Autodesk Inventor part; units mm, degrees
ref_plane "YZ Plane" through (0, 0, 0) normal (1, 0, 0) x (0, 1, 0)
ref_plane "XZ Plane" through (0, 0, 0) normal (0, 1, 0) x (-1, 0, 0)
ref_plane "XY Plane" through (0, 0, 0) normal (0, 0, 1) x (1, 0, 0)
sketch "Sketch1" plane through (0, 0, 0) normal (0, 1, 0) x (-1, 0, 0)
  arc A0 (2.8605, 1.9692) -> (1.9692, 2.8605) centre (2.4696, 2.4696) ccw
  line L0 (1.3405, 2.2319) -> (1.9692, 2.8605)
  arc A1 (1.3405, 2.2319) -> (-1.3405, 2.2319) centre (0, 0) ccw
  line L1 (-1.9692, 2.8605) -> (-1.3405, 2.2319)
  arc A2 (-1.9692, 2.8605) -> (-2.8605, 1.9692) centre (-2.4696, 2.4696) ccw
  line L2 (-2.2319, 1.3405) -> (-2.8605, 1.9692)
  arc A3 (-2.2319, 1.3405) -> (-2.2319, -1.3405) centre (0, 0) ccw
  line L3 (-2.8605, -1.9692) -> (-2.2319, -1.3405)
  arc A4 (-2.8605, -1.9692) -> (-1.9692, -2.8605) centre (-2.4696, -2.4696) ccw
  line L4 (-1.3405, -2.2319) -> (-1.9692, -2.8605)
  arc A5 (-1.3405, -2.2319) -> (1.3405, -2.2319) centre (0, 0) ccw
  line L5 (1.9692, -2.8605) -> (1.3405, -2.2319)
  arc A6 (1.9692, -2.8605) -> (2.8605, -1.9692) centre (2.4696, -2.4696) ccw
  line L6 (2.2319, -1.3405) -> (2.8605, -1.9692)
  arc A7 (2.2319, -1.3405) -> (2.2319, 1.3405) centre (0, 0) ccw
  line L7 (2.8605, 1.9692) -> (2.2319, 1.3405)
  arc A8 (-4.5172, 1.6401) -> (-5.4471, 3.8852) centre (-7.6922, 1.6401) ccw
  line L8 (-8.7558, 7.1939) -> (-5.4471, 3.8852)
  arc A9 (-8.7558, 7.1939) -> (-10.4905, 6.4753) centre (-9.4743, 6.4753) ccw
  line L9 (-10.4905, -6.4748) -> (-10.4905, 6.4753)
  arc A10 (-10.4905, -6.4748) -> (-8.7558, -7.1933) centre (-9.4743, -6.4748) ccw
  line L10 (-5.4471, -3.8846) -> (-8.7558, -7.1933)
  arc A11 (-5.4471, -3.8846) -> (-4.5172, -1.6396) centre (-7.6922, -1.6396) ccw
  line L11 (-4.5172, 1.6401) -> (-4.5172, -1.6396)
  arc A12 (1.6396, 4.5172) -> (3.8846, 5.4471) centre (1.6396, 7.6922) ccw
  line L12 (3.8846, 5.4471) -> (7.1933, 8.7558)
  arc A13 (7.1933, 8.7558) -> (6.4748, 10.4905) centre (6.4748, 9.4743) ccw
  line L13 (6.4748, 10.4905) -> (4.356, 10.4905)
  arc A14 (4.356, 12.7003) -> (4.356, 10.4905) centre (4.356, 11.5954) ccw
  line L14 (4.356, 12.7003) -> (10.5919, 12.7003)
  arc A15 (12.7001, 10.5921) -> (10.5919, 12.7003) centre (10.5919, 10.5921) ccw
  line L15 (12.7001, 10.5921) -> (12.7001, 4.3562)
  arc A16 (10.4903, 4.3562) -> (12.7001, 4.3562) centre (11.5952, 4.3562) ccw
  line L16 (10.4903, 4.3562) -> (10.4903, 6.475)
  arc A17 (10.4903, 6.475) -> (8.7555, 7.1936) centre (9.4741, 6.475) ccw
  line L17 (8.7555, 7.1936) -> (5.4468, 3.8849)
  arc A18 (5.4468, 3.8849) -> (4.5169, 1.6399) centre (7.6919, 1.6399) ccw
  line L18 (4.5169, 1.6399) -> (4.5169, -1.6396)
  arc A19 (4.5169, -1.6396) -> (5.4468, -3.8846) centre (7.6919, -1.6396) ccw
  line L19 (5.4468, -3.8846) -> (8.7555, -7.1933)
  arc A20 (8.7555, -7.1933) -> (10.4903, -6.4748) centre (9.4741, -6.4748) ccw
  line L20 (10.4903, -6.4748) -> (10.4903, -4.356)
  arc A21 (12.7001, -4.356) -> (10.4903, -4.356) centre (11.5952, -4.356) ccw
  line L21 (12.7001, -4.356) -> (12.7001, -10.5919)
  arc A22 (10.5919, -12.7001) -> (12.7001, -10.5919) centre (10.5919, -10.5919) ccw
  line L22 (10.5919, -12.7001) -> (4.356, -12.7001)
  arc A23 (4.356, -10.4903) -> (4.356, -12.7001) centre (4.356, -11.5952) ccw
  line L23 (4.356, -10.4903) -> (6.475, -10.4903)
  arc A24 (6.475, -10.4903) -> (7.1936, -8.7555) centre (6.475, -9.4741) ccw
  line L24 (7.1936, -8.7555) -> (3.8846, -5.4465)
  arc A25 (3.8846, -5.4465) -> (1.6396, -4.5166) centre (1.6396, -7.6916) ccw
  line L25 (1.6396, -4.5166) -> (-1.6396, -4.5166)
  arc A26 (-1.6396, -4.5166) -> (-3.8846, -5.4465) centre (-1.6396, -7.6916) ccw
  line L26 (-3.8846, -5.4465) -> (-7.1936, -8.7555)
  arc A27 (-7.1936, -8.7555) -> (-6.475, -10.4903) centre (-6.475, -9.4741) ccw
  line L27 (-6.475, -10.4903) -> (-4.3562, -10.4903)
  arc A28 (-4.3562, -12.7001) -> (-4.3562, -10.4903) centre (-4.3562, -11.5952) ccw
  line L28 (-4.3562, -12.7001) -> (-10.5919, -12.7001)
  arc A29 (-12.7001, -10.5919) -> (-10.5919, -12.7001) centre (-10.5919, -10.5919) ccw
  line L29 (-12.7001, -10.5919) -> (-12.7001, 10.5921)
  arc A30 (-10.5919, 12.7003) -> (-12.7001, 10.5921) centre (-10.5919, 10.5921) ccw
  line L30 (-10.5919, 12.7003) -> (-4.3562, 12.7003)
  arc A31 (-4.3562, 10.4905) -> (-4.3562, 12.7003) centre (-4.3562, 11.5954) ccw
  line L31 (-4.3562, 10.4905) -> (-6.475, 10.4905)
  arc A32 (-6.475, 10.4905) -> (-7.1936, 8.7558) centre (-6.475, 9.4743) ccw
  line L32 (-7.1936, 8.7558) -> (-3.8849, 5.4471)
  arc A33 (-3.8849, 5.4471) -> (-1.6399, 4.5172) centre (-1.6399, 7.6922) ccw
  line L33 (-1.6399, 4.5172) -> (1.6396, 4.5172)
  point P0 (0, 0)
  dimension "d36" = 8.1835
  dimension "d81" = 1.0162
  dimension "d82" = 3.175
  dimension "d95" = 8.1832
  dimension "d96" = 17.2172
  dimension "d97" = 23.1906
  dimension "d98" = 25.4002
  dimension "d100" = 8.1832
  dimension "d101" = 2.2092
  dimension "d104" = 2.2091
  dimension "d131" = 1.1049
  dimension "d132" = 2.1082
  dimension "d133" = 0.635
  dimension "d134" = 2.6035
  dimension "d135" = 2.6035
  dimension "d136" = 2.6035
  dimension "d137" = 2.6035
  dimension "d138" = 45
  dimension "d139" = 45
  dimension "d140" = 45
  dimension "d141" = 45
  dimension "d142" = 45
  dimension "d143" = 25.4004
  dimension "d144" = 0.4742
  dimension "d145" = 1.7347
  dimension "d146" = 0.4744
  dimension "d147" = 1.7349
  dimension "d148" = 12.7001
  dimension "d149" = 12.7003
  dimension "d150" = 1.1046
  dimension "d151" = 1.1048
  dimension "d152" = 0.6303
  dimension "d153" = 0.6303
  dimension "d154" = 0.6303
  dimension "d155" = 0.6303
  dimension "d156" = 8.3441
  dimension "d157" = 17.0563
  dimension "d158" = 8.3441
  dimension "d159" = 8.3441
  dimension "d160" = 9.8396
  dimension "d161" = 9.8396
  dimension "d162" = 10.2305
  dimension "d163" = 10.2305
  dimension "d164" = 10.4682
  dimension "d165" = 10.4682
  dimension "d166" = 14.6692
  dimension "d167" = 14.6692
  dimension "d168" = 15.1696
  dimension "d169" = 15.1696
  dimension "d170" = 17.0563
  dimension "d171" = 17.0563
extrude "Extrusion1" add sketch "Sketch1" along normal mid plane 25.4
properties part number "1003-S-BLACK-FB" material "6105-T5"
The listing builds one solid part. Answer for the finished solid, in the listing's coordinates (mm). A direction names the side the tool comes from. Coordinates: 2 decimals unless noted, no trailing zeros. Write each loop counter-clockwise with the first axis right and the second up, starting at its lowest first coordinate (ties: lowest second). Pieces come first, ordered by that corner, then holes.
Q1. Section D-D, the plane y = 10.25 is taken. Give the number of separate pieces and of enclosed holes in the cut face, then the cut area to 3 significant figures.
Returned:
separate pieces: 1
enclosed holes: 2
area: 295 mm2
Q2. Given P1, Ø1, axis at x = 0, y = 2.5, coming from the +Z side; P2, Ø1, axis at x = -2.47, z = -2.47, coming from the -Y side; P3, Ø1.6, axis at y = 2.5, z = 0, coming from the -X side; P4, Ø1.6, axis at x = 0, y = -5, coming from the -Z side, each flat-ended and moving along its own axis, determine where each tip first touches the part or whether it passes through.
Returned:
P1: stops at z = 4.52
P2: passes through
P3: stops at x = -4.52
P4: stops at z = -4.52
Q3. Section C-C, the plane x = -5 is taken. Write down the section's boundary in (y, z), then the cut area to 3 significant figures.
Returned:
outline: (-12.7, -12.7) - (12.7, -12.7) - (12.7, -10.49) - (-12.7, -10.49) - close; (-12.7, -6.56) - (12.7, -6.56) - (12.7, -3.32) - (-12.7, -3.32) - close; (-12.7, 3.32) - (12.7, 3.32) - (12.7, 6.56) - (-12.7, 6.56) - close; (-12.7, 10.49) - (12.7, 10.49) - (12.7, 12.7) - (-12.7, 12.7) - close
area: 277 mm2
Q4. The mould has two halves that part along Z. Classify faces 3 (the cylindrical face through (2.871, -0.178, -4.765)), 4 (the flat face through (-8, 0, -12.7)), 5 (the cylindrical face through (-4.752, -0.178, 2.839)), 6 (the flat face through (-7, 0, 12.7)): released by +Z, released by -Z, zero draft, split by the parting line, or undercut.
Returned:
face 3: undercut
face 4: released by -Z
face 5: undercut
face 6: released by +Z
Q5. Section B-B, the plane z = 11 is taken. Write down the section's boundary in (x, y), then the cut area to 3 significant figures.
Returned:
outline: (-12.66, -12.7) - (-3.43, -12.7) - (-3.43, 12.7) - (-12.66, 12.7) - close; (3.43, -12.7) - (12.66, -12.7) - (12.66, 12.7) - (3.43, 12.7) - close
area: 469 mm2
Q6. Find the intervals of material crossed by line 1 along Z through (x, y) = (-4.25, 11.5) (1 decimal); line 2 along Z through (x, y) = (-4, 5); line 3 along X through (y, z) = (-3.25, -5.25), in increasing order.
Returned:
line 1: z = -12.7 to -10.5, -5.8 to 5.8, 10.5 to 12.7
line 2: z = -12.64 to -10.55, -5.56 to 5.56, 10.55 to 12.64
line 3: x = -12.7 to -10.49, -6.81 to -3.67, 3.67 to 6.81, 10.49 to 12.7
Q7. Section A-A, the plane x = -11 is taken. Write down the section's boundary in (y, z).
Returned:
outline: (-12.7, -12.66) - (12.7, -12.66) - (12.7, -3.43) - (-12.7, -3.43) - close; (-12.7, 3.43) - (12.7, 3.43) - (12.7, 12.66) - (-12.7, 12.66) - close
Q8. Which of the six approach directions +Z, -Z, +X, -X, +Y, -Y give full straight-line access (tool end or side, diameter ignored) to faces 1 (the cylindrical face through (4.752, -0.178, -2.838)), 2 (the flat face through (8, 0, 12.7))?
Returned:
face 1: +Y, -Y
face 2: +Z, +X, -X, +Y, -Y
